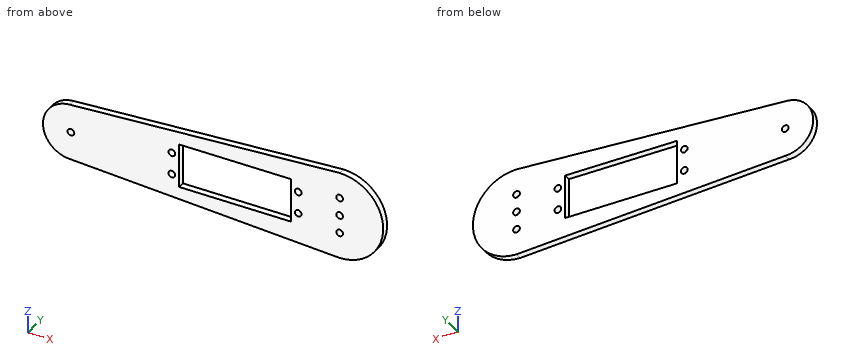
Autodesk Inventor part; units mm, degrees
ref_plane "YZ Plane" through (0, 0, 0) normal (1, 0, 0) x (0, 1, 0)
ref_plane "XZ Plane" through (0, 0, 0) normal (0, 1, 0) x (-1, 0, 0)
ref_plane "XY Plane" through (0, 0, 0) normal (0, 0, 1) x (1, 0, 0)
sketch "Boceto1" plane through (0, 0, 0) normal (0, 1, 0) x (-1, 0, 0)
  arc A0 (120.2602, -12.5039) -> (120.5206, 12.4893) centre (120.13, -0.0046) ccw
  line L0 (21.75, -9.75) -> (71.75, -9.75)
  line L1 (71.75, -9.75) -> (71.75, 9.75)
  line L2 (71.75, 9.75) -> (21.75, 9.75)
  line L3 (21.75, 9.75) -> (21.75, -9.75)
  circle A1 centre (75, 4.875) radius 1.5
  circle A2 centre (75, -4.875) radius 1.5
  circle A3 centre (18.5, 4.875) radius 1.5
  circle A4 centre (18.5, -4.875) radius 1.5
  line L4 (0, 19.5) -> (120.5119, 12.4874)
  line L5 (0, -19.5) -> (119.9998, -12.5039)
  arc A5 (0, 19.5) -> (0, -19.5) centre (0, 0) ccw
  circle A6 centre (120.13, -0.0046) radius 1.5
  circle A7 centre (0, 0) radius 1.5
  circle A8 centre (0, -8) radius 1.5
  circle A9 centre (0, 8) radius 1.5
  line L6 (120.2602, -12.5039) -> (119.9998, -12.5039)
  line L7 (120.5206, 12.4893) -> (120.5119, 12.4874)
  dimension "d107" = 3
  dimension "d108" = 3
  dimension "d110" = 3
  dimension "d112" = 3
extrude "Extrusión1" add sketch "Boceto1" along normal blind 3
properties part number "brazo1"
Build history of the part. All positions in model axes, mm. Give positions to 0.01 mm unless a question says otherwise; leave off trailing zeros. Loops run counter-clockwise (first coordinate to the right, second up) from the corner with the lowest first, then second, coordinate; pieces in that order, holes last. Notation, with made-up numbers: (73, 42.25) -> (82, 42.25) arc R35 ccw to (82, 76.25) -> close; hole circle Ø8 at (44, 12). An arc over 180 degrees is marked (long way). Answer in a Markdown table with one row per item.
Item 1: Slice it at D-D on z = -17. Write the cut outline in (x, y), plus the area to 3 significant figures.
Findings below:
| item | result |
|---|---|
| outline | (-42.88, 0) -> (9.55, 0) -> (9.55, 3) -> (-42.88, 3) -> close |
| area | 157 mm² |
Item 2: Probe line 1 along Z through (x, y) = (0, 2.2); line 2 along Z through (x, y) = (-120.13, 2.1); line 3 along X through (y, z) = (2.4, -5.5). List the from-to ranges inside material, lowest first. Write a range as [from, to].
Findings below:
| item | result |
|---|---|
| line 1 | z = [-19.5, -9.5], [-6.5, -1.5], [1.5, 6.5], [9.5, 19.5] |
| line 2 | z = [-12.5, -1.5], [1.5, 12.51] |
| line 3 | x = [-131.36, -76.36], [-73.64, -71.75], [-21.75, -19.86], [-17.14, 18.71] |
Item 3: Flat gauge pins, fed straight in: P1, Ø1.5, axis at y = 0.5, z = -6, coming from the -X side; P2, Ø1.5, axis at y = 1.5, z = 2.5, coming from the -X side; P3, Ø4, axis at x = -41, z = 7, coming from the +Y side; P4, Ø1, axis at y = 1.5, z = 8, coming from the -X side. Where does each tip first touch, or does it go through?
Findings below:
| item | result |
|---|---|
| P1 | stops at x = -131.48 |
| P2 | stops at x = -132.51 |
| P3 | passes through |
| P4 | stops at x = -130.13 |
Item 4: Slice it at A-A on z = -8. Write the cut outline in (x, y), plus the area to 3 significant figures.
Findings below:
| item | result |
|---|---|
| outline | (-129.74, 0) -> (-71.75, 0) -> (-71.75, 3) -> (-129.74, 3) -> close; (-21.75, 0) -> (-1.5, 0) -> (-1.5, 3) -> (-21.75, 3) -> close; (1.5, 0) -> (17.78, 0) -> (17.78, 3) -> (1.5, 3) -> close |
| area | 284 mm² |
Item 5: Slice it at B-B on y = 0.6. Give the number of separate pieces and of enclosed holes in the cut face, plus the area to 3 significant figures.
Findings below:
| item | result |
|---|---|
| separate pieces | 1 |
| enclosed holes | 9 |
| area | 3,660 mm² |
Item 6: Slice it at C-C on x = -18.5. Write the cut outline in (y, z) (3 decimals).
Findings below:
| item | result |
|---|---|
| outline | (0, -18.421) -> (3, -18.421) -> (3, -6.375) -> (0, -6.375) -> close; (0, -3.375) -> (3, -3.375) -> (3, 3.375) -> (0, 3.375) -> close; (0, 6.375) -> (3, 6.375) -> (3, 18.423) -> (0, 18.423) -> close |
